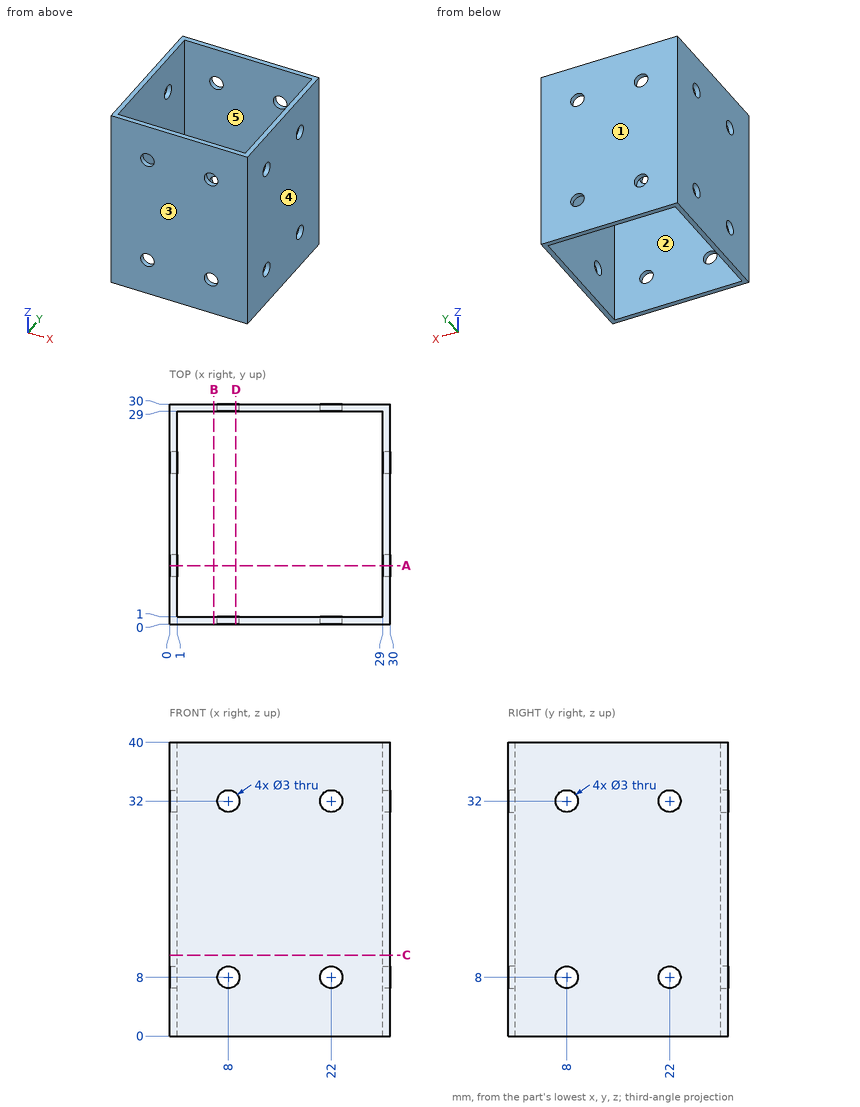
Job drawing, mm, ordinate dimensions from the low corner. One solid piece. A direction names the side the tool comes from. Give positions to 0.01 mm unless a question says otherwise; leave off trailing zeros. Order: outer loops, then holes, each group sorted by start corner. A loop starts at its lowest first (then second) coordinate and runs counter-clockwise, first axis right, second up. Notation, with made-up numbers: (88, -29.75) - (126, -29.75) arc R29 cw to (126, -0.75) - close; hole circle Ø9 at (64.5, 0). An arc over 180 degrees is marked (long way). Answer in a Markdown table with one row per item.
1. Probe probe 1 along Y at (x, z) = (29.45, 32); probe 2 along X at (y, z) = (19.5, 12). List the from-to ranges inside material, lowest first. Write a range as [from, to].
Data:
| item | result |
|---|---|
| probe 1 | y = [0, 6.5], [9.5, 20.5], [23.5, 30] |
| probe 2 | x = [0, 1], [29, 30] |
2. Saw through at B-B, the plane x = 6. Give the cut face in (y, z).
Data:
| item | result |
|---|---|
| outline | (0, 0) - (1, 0) - (1, 40) - (0, 40) - close; (29, 0) - (30, 0) - (30, 40) - (29, 40) - close |
3. Pull direction Y, two halves, no side cores. Call the marked faces 1, 2 and 3: pulls with the +Y half, pulls with the -Y half, needs draft (parallel to the pull), parting line crosses it, or undercut.
Data:
| item | result |
|---|---|
| face 1 | pulls with the +Y half |
| face 2 | undercut |
| face 3 | pulls with the -Y half |
4. Saw through at C-C, the plane z = 11. Give the cut face in (x, y), plus the area to 3 significant figures.
Data:
| item | result |
|---|---|
| outline | (0, 0) - (30, 0) - (30, 30) - (0, 30) - close; hole (1, 1) - (29, 1) - (29, 29) - (1, 29) - close |
| area | 116 mm² |
5. Flat gauge pin, fed straight in: pin 1 (10 mm diameter, centred on x = 23.5, y = 18.5, fed in from -Z). Where does the tip first touch, or does it go through?
Data:
| item | result |
|---|---|
| pin 1 | passes through |
6. Saw through at A-A, the plane y = 8. Give the cut face in (x, z), plus the area to 3 significant figures.
Data:
| item | result |
|---|---|
| outline | (0, 0) - (1, 0) - (1, 6.5) - (0, 6.5) - close; (0, 9.5) - (1, 9.5) - (1, 30.5) - (0, 30.5) - close; (0, 33.5) - (1, 33.5) - (1, 40) - (0, 40) - close; (29, 0) - (30, 0) - (30, 6.5) - (29, 6.5) - close; (29, 9.5) - (30, 9.5) - (30, 30.5) - (29, 30.5) - close; (29, 33.5) - (30, 33.5) - (30, 40) - (29, 40) - close |
| area | 68.0 mm² |
7. Saw through at D-D, the plane x = 9. Give the cut face in (y, z).
Data:
| item | result |
|---|---|
| outline | (0, 0) - (1, 0) - (1, 6.88) - (0, 6.88) - close; (0, 9.12) - (1, 9.12) - (1, 30.88) - (0, 30.88) - close; (0, 33.12) - (1, 33.12) - (1, 40) - (0, 40) - close; (29, 0) - (30, 0) - (30, 6.88) - (29, 6.88) - close; (29, 9.12) - (30, 9.12) - (30, 30.88) - (29, 30.88) - close; (29, 33.12) - (30, 33.12) - (30, 40) - (29, 40) - close |
8. Tool access for the marked faces 4 and 5: list every direction of +Z, -Z, +X, -X, +Y, -Y with a clear straight run to the whole face (end or side of a thin tool).
Data:
| item | result |
|---|---|
| face 4 | +Z, -Z, +X, +Y, -Y |
| face 5 | +Z, -Z |
